```python
from build123d import *

# Parameters (mm, degrees)
RESSALTO_EXTRUS_O1_DEPTH = 178
ESBO_O2_R                = 8
CORTE_EXTRUS_O1_DEPTH    = 655
RESSALTO_EXTRUS_O2_DEPTH = 22
RESSALTO_EXTRUS_O3_DEPTH = 22
ESBO_O5_W                = 8
ESBO_O5_H                = 32.976988492
CORTE_EXTRUS_O2_DEPTH    = 89
CHANFRO1_SIZE            = 50
CHANFRO1_SIZE2           = 8.816349035
CORTE_EXTRUS_O3_DEPTH    = 108
CHANFRO2_SIZE            = 3
ESBO_O7_R                = 8
CORTE_EXTRUS_O4_DEPTH    = 89


with BuildPart() as part:
    # Esboço1 → Ressalto-extrusão1 (new, symmetric)
    with BuildSketch(Plane.XY):
        Polygon((-19, 0), (19, 0), (19, 6), (24, 6), (24, -30), (-24, -30), (-24, 6), (-19, 6), align=None)
    extrude(amount=RESSALTO_EXTRUS_O1_DEPTH, both=True)

    # Esboço2 → Corte-extrusão1 (cut)
    with BuildSketch(Plane(origin=(24, 0, 0), x_dir=(0, 0, -1), z_dir=(1, 0, 0))):
        with Locations(Location((-148, -15, 0), (0, 0, 90))):
            Circle(ESBO_O2_R)
        with Locations(Location((148, -15, 0), (0, 0, 90))):
            Circle(ESBO_O2_R)
    extrude(amount=-CORTE_EXTRUS_O1_DEPTH, mode=Mode.SUBTRACT)

    # Esboço3 → Ressalto-extrusão2 (add)
    with BuildSketch(Plane.XY.offset(178)):
        Polygon((-24, 6), (-24, -30), (24, -30), (24, 6), (19, 6), (19, 0), (-19, 0), (-19, 6), align=None)
    extrude(amount=RESSALTO_EXTRUS_O2_DEPTH)

    # Esboço4 → Ressalto-extrusão3 (add)
    with BuildSketch(Plane(origin=(0, 0, -178), x_dir=(-1, 0, 0), z_dir=(0, 0, -1))):
        Polygon((24, -30), (24, 6), (19, 6), (19, 0), (-19, 0), (-19, 6), (-24, 6), (-24, -30), align=None)
    extrude(amount=RESSALTO_EXTRUS_O3_DEPTH)

    # Esboço5 → Corte-extrusão2 (cut)
    with BuildSketch(Plane(origin=(24, 0, 0), x_dir=(0, 0, -1), z_dir=(1, 0, 0))):
        with Locations((104, -40.488494246)):
            Rectangle(ESBO_O5_W, ESBO_O5_H)
    extrude(amount=-CORTE_EXTRUS_O2_DEPTH, mode=Mode.SUBTRACT)

    # Chanfro1
    chanfro1_edges = [part.edges().sort_by_distance(p)[0] for p in [
        (0, 0, 200),
        (0, 0, -200),
    ]]
    chanfro1_side = [part.faces().sort_by_distance(p)[0] for p in [
        (0, 0, 0),
    ]]
    chamfer(chanfro1_edges, length=CHANFRO1_SIZE, length2=CHANFRO1_SIZE2, reference=chanfro1_side[0])

    # Esboço6 → Corte-extrusão3 (cut)
    with BuildSketch(Plane(origin=(24, 0, 0), x_dir=(0, 0, -1), z_dir=(1, 0, 0))):
        Polygon((-135.211980872, 8.700086435), (-200, 6), (-201.041889066, -2.907502517), align=None)
        Polygon((200, 6), (201.041889066, -2.907502517), (135.211980872, 8.700086435), align=None)
    extrude(amount=-CORTE_EXTRUS_O3_DEPTH, mode=Mode.SUBTRACT)

    # Chanfro2
    chanfro2_edges = [part.edges().sort_by_distance(p)[0] for p in [
        (24, -30, 50),
        (-24, -30, 50),
        (24, -30, -154),
        (-24, -30, -154),
    ]]
    chamfer(chanfro2_edges, length=CHANFRO2_SIZE)

    # Esboço7 → Corte-extrusão4 (cut)
    with BuildSketch(Plane(origin=(24, 0, 0), x_dir=(0, 0, -1), z_dir=(1, 0, 0))):
        with Locations(Location((0, -15, 0), (0, 0, 90))):
            Circle(ESBO_O7_R)
    extrude(amount=-CORTE_EXTRUS_O4_DEPTH, mode=Mode.SUBTRACT)


solid = part.part
```
Geometry check sheet. Reference: the model listing, model coordinates, mm. A direction names the side the tool comes from. Coordinates: 2 decimals unless noted, no trailing zeros. Order: outer loops, then holes, each group sorted by start corner. A loop starts at its lowest first (then second) coordinate and runs counter-clockwise, first axis right, second up. Notation, with made-up numbers: (63, 61) - (85, 61) arc R31 cw to (85, 90) - close; hole circle Ø11 at (68.5, 20.25). An arc over 180 degrees is marked (long way). Answer in a Markdown table with one row per item. Add a question column.
1. Section check B-B (x = 10). Enter the section's corners in (y, z).
2. Access from +Z, -Z, +X, -X, +Y, -Y to the whole of each face (thin tool, end or side, straight path). Record for faces 1 (the face through (0.27, -4.47, 175.35)), 2 (the face through (-0.27, -4.47, -175.35)), 3 (the face through (0, 0, 2)).
3. Section check C-C (z = 0). Enter the section's corners in (x, y), plus the area to 3 significant figures.
4. Section check A-A (y = -15). Enter the section's corners in (x, z), plus the area to 3 significant figures.
5. Draft check along Z on faces 4 (the face through (19, 2, 3)), 5 (the face through (-21.465, 1.577, -175.609)), 6 (the face through (0, -24, -104)). Enter one of: +Z half, -Z half, draft (parallel to the pull), parting line (faces both ways), or undercut.
6. Gauge pin test, flat ends, axial feed: pin 1 Ø13 at (y, z) = (-15, 0) entering from -X; pin 2 Ø5 at (x, z) = (-11, -118.5) entering from +Y. Record the tip position at first contact, or that the pin passes through.
7. Material ranges on L1, parallel to Z at x = -12, y = -15; L2, parallel to X at y = 4.5, z = 102; L3, parallel to Z at x = 11, y = -10.5, recorded low to high. Write a range as [from, to].
Data:
| question | item | result |
|---|---|---|
| 1 | outline | (-30, -200) - (-8.82, -200) - (0, -150) - (0, 150) - (-8.82, 200) - (-30, 200) - (-30, -100) - (-24, -100) - (-24, -108) - (-30, -108) - close; hole circle Ø16 at (-15, -148); hole circle Ø16 at (-15, 0); hole circle Ø16 at (-15, 148) |
| 2 | face 1 | +Z, +Y |
| 2 | face 2 | -Z, +Y |
| 2 | face 3 | +Z, -Z, +Y |
| 3 | outline | (-24, -27) - (-21, -30) - (21, -30) - (24, -27) - (24, -23) - (-24, -23) - close; (-24, -7) - (24, -7) - (24, 6) - (19, 6) - (19, 0) - (-19, 0) - (-19, 6) - (-24, 6) - close |
| 3 | area | 723 mm² |
| 4 | outline | (-24, -200) - (24, -200) - (24, -156) - (-24, -156) - close; (-24, -140) - (24, -140) - (24, -8) - (-24, -8) - close; (-24, 8) - (24, 8) - (24, 140) - (-24, 140) - close; (-24, 156) - (24, 156) - (24, 200) - (-24, 200) - close |
| 4 | area | 16,900 mm² |
| 5 | face 4 | draft |
| 5 | face 5 | -Z half |
| 5 | face 6 | undercut |
| 6 | pin 1 | passes through |
| 6 | pin 2 | stops at y = 0 |
| 7 | L1 | z = [-200, -156], [-140, -8], [8, 140], [156, 200] |
| 7 | L2 | x = [-24, -19], [19, 24] |
| 7 | L3 | z = [-200, -154.61], [-141.39, -6.61], [6.61, 141.39], [154.61, 200] |
